```python
from build123d import *

# Parameters (mm, degrees)
SKETCH1_W          = 3.5
SKETCH1_H          = 8
CUT_EXTRUDE1_DEPTH = 2


# Read off the part's stored shape, not the designer's step: M6x1.0 Machine Threads Stud1
with BuildPart() as part:
    # Sketch1 → Revolve1 (revolve)
    with BuildSketch(Plane.XY, mode=Mode.PRIVATE) as revolve1_sk:
        with Locations((1.75, -5.693638198)):
            Rectangle(SKETCH1_W, SKETCH1_H)
        Polygon((5.193638198, 0), (0, 0), (0, -1.693638198), (3.5, -1.693638198), align=None)
    revolve(revolve1_sk.sketch.rotate(Axis((0, 39.805194805, 0), (0, -1, 0)), 90), axis=Axis((0, 39.805194805, 0), (0, -1, 0)))

    # Sketch2 → Cut-Extrude1 (cut)
    with BuildSketch(Plane(origin=(0, 0, 0), x_dir=(1, 0, 0), z_dir=(0, 1, 0))):
        Polygon((0.577350269, -1), (1.154700538, 0), (0.577350269, 1), (-0.577350269, 1), (-1.154700538, 0), (-0.577350269, -1), align=None)
    extrude(amount=-CUT_EXTRUDE1_DEPTH, mode=Mode.SUBTRACT)

    # M6x1.0 Machine Threads Stud1 outline → M6x1.0 Machine Threads Stud1 (revolve, cut)
    with BuildSketch(Plane.XY):
        Polygon((2.4455, -9.693638198), (3.5, -9.693638198), (3.5, -1.693638198), (3, -1.693638198), (3, -9.139138198), align=None)
    revolve(axis=Axis((0, 0, 0), (0, 1, 0)), mode=Mode.SUBTRACT)


solid = part.part
```
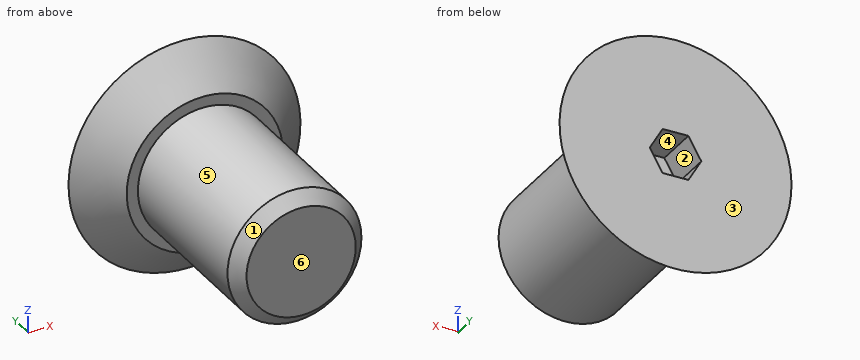
The listing builds one solid part. Answer for the finished solid, in the listing's coordinates (mm). Face numbers are marked on the shaded views. A direction names the side the tool comes from. Round coordinates to 2 decimals unless told otherwise and drop trailing zeros. Loops run counter-clockwise (first coordinate to the right, second up) from the corner with the lowest first, then second, coordinate; pieces in that order, holes last.
Q1. Find the intervals of material crossed by line 1 (Y direction, x = 1.5, z = 3.75); line 2 (Y direction, x = 0.75, z = 3.25); line 3 (X direction, y = -8.5, z = 2.75), in increasing order.
Q2. Section B-B, the plane x = 0 is taken. Determine the outline of the cut face in (y, z).
Q3. For a pull along Z with two mould halves and no side action, classify the marked faces 1, 2 and 3 as released by +Z, released by -Z, zero draft, split by the parting line, or undercut.
Q4. Which of the six approach directions +Z, -Z, +X, -X, +Y, -Y give full straight-line access (tool end or side, diameter ignored) to the marked faces 4, 5 and 6?
Q5. Given pin 1 Ø0.9 at (x, y) = (0, -0.5) entering from +Z; pin 2 Ø5 at (y, z) = (-5.5, 3) entering from -X; pin 3 Ø3 at (x, z) = (-4, 3.5) entering from -Y, each flat-ended and moving along its own axis, determine where each tip first touches the part or whether it passes through.
Q6. Section A-A, the plane y = -0.25 is taken. Determine the outline of the cut face in (x, z).
Q7. Section C-C, the plane y = -3 is taken. Determine the outline of the cut face in (x, z).
Completed:
1. line 1: y = -1.15 to 0
1. line 2: y = -1.69 to 0
1. line 3: x = -1.2 to 1.2
2. outline: (-9.69, -2.45) - (-9.14, -3) - (-1.69, -3) - (-1.69, -3.5) - (0, -5.19) - (0, -1) - (-2, -1) - (-2, 1) - (0, 1) - (0, 5.19) - (-1.69, 3.5) - (-1.69, 3) - (-9.14, 3) - (-9.69, 2.45) - close
3. face 1: split by the parting line
3. face 2: undercut
3. face 3: zero draft
4. face 4: +Y
4. face 5: -Y
4. face 6: +Z, -Z, +X, -X, -Y
5. pin 1: stops at z = 5.14
5. pin 2: stops at x = -2.96
5. pin 3: stops at y = -1.38
6. outline: circle Ø9.89 at (0, 0); hole (-1.15, 0) - (-0.58, -1) - (0.58, -1) - (1.15, 0) - (0.58, 1) - (-0.58, 1) - close
7. outline: circle Ø6 at (0, 0)
